Verification items for this drawing (mm, ordinates from the low corner). Round coordinates to 2 decimals unless told otherwise and drop trailing zeros. Order: outer loops, then holes, each group sorted by start corner. A loop starts at its lowest first (then second) coordinate and runs counter-clockwise, first axis right, second up. Notation, with made-up numbers: (78.25, -24) -> (106.25, -24) arc R35 cw to (106.25, 12) -> close; hole circle Ø1 at (-34, 56.25). An arc over 180 degrees is marked (long way). Answer in a Markdown table with one row per item. Add a question column.
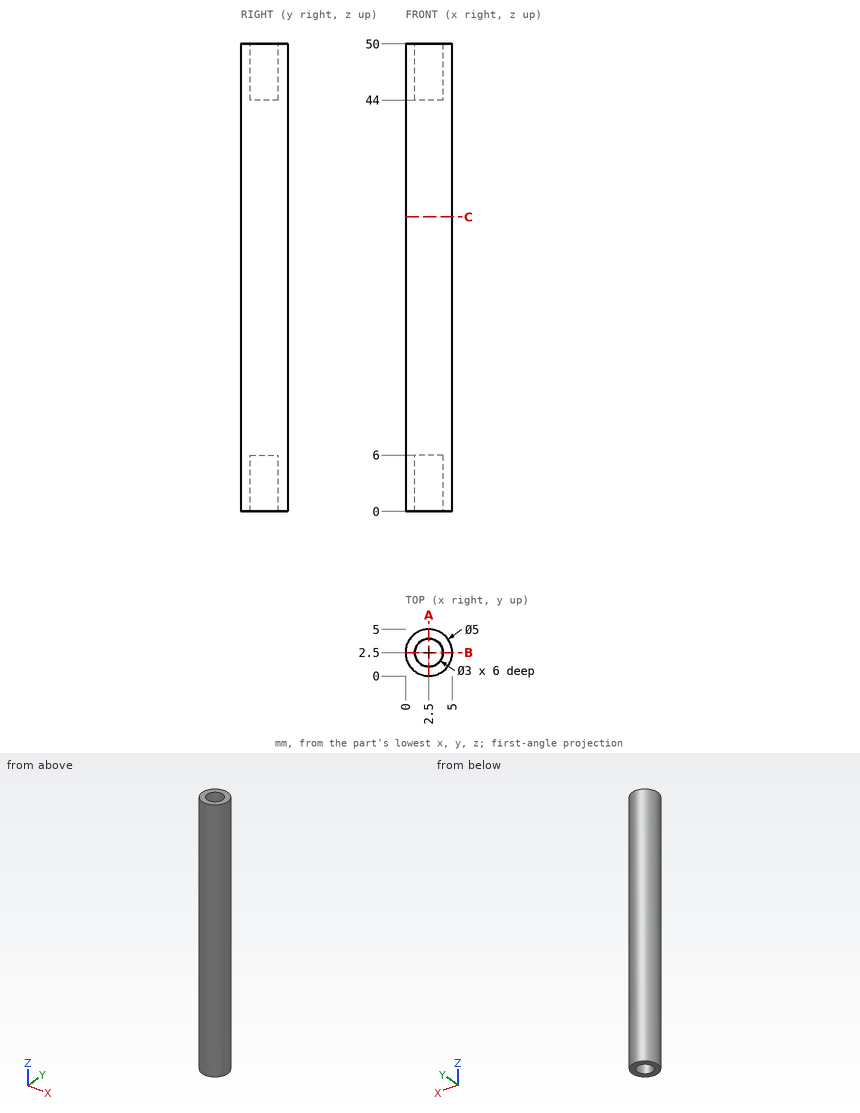
1) Cross-section at C-C, the plane z = 31.5. Record the boundary of the cut face in (x, y), and give its area (3 significant figures).
2) Depth check by flat-ended pin: P1, Ø1.5, axis at x = 3, z = 43, coming from the -Y side; P2, Ø1, axis at x = 0.5, z = 18, coming from the +Y side; P3, Ø0.9, axis at x = 3, y = 2, coming from the +Z side; P4, Ø1.5, axis at x = 2, y = 3, coming from the -Z side. Enter the tip coordinate at first touch or a pass-through.
3) Thickness scan on L1, parallel to Y at x = 2.5, z = 46.45; L2, parallel to Y at x = 4.5, z = 15.5; L3, parallel to Z at x = 2.45, y = 2.25. Record the ranges inside material, lowest first. Write a range as [from, to].
4) Cross-section at A-A, the plane x = 2.5. Record the boundary of the cut face in (y, z).
Results below:
| question | item | result |
|---|---|---|
| 1 | outline | circle Ø5 at (2.5, 2.5) |
| 1 | area | 19.6 mm² |
| 2 | P1 | y = 0 |
| 2 | P2 | y = 4.5 |
| 2 | P3 | z = 44 |
| 2 | P4 | z = 6 |
| 3 | L1 | [0, 1], [4, 5] |
| 3 | L2 | [1, 4] |
| 3 | L3 | [6, 44] |
| 4 | outline | (0, 0) -> (1, 0) -> (1, 6) -> (4, 6) -> (4, 0) -> (5, 0) -> (5, 50) -> (4, 50) -> (4, 44) -> (1, 44) -> (1, 50) -> (0, 50) -> close |
